Can you work these out from the model? Positions are in its coordinate system, mm. A direction names the side the tool comes from. Give positions to 0.01 mm unless a question says otherwise; leave off trailing zeros. Write each loop counter-clockwise with the first axis right and the second up, starting at its lowest first coordinate (ties: lowest second). Pieces come first, ordered by that corner, then holes. Notation, with made-up numbers: (23.5, -35) -> (73.5, -35) arc R11 cw to (73.5, -27) -> close; hole circle Ø1 at (73, 65.25). An arc over 180 degrees is marked (long way). One line per item, written item: value.
from build123d import *

# Parameters (mm, degrees)
SKETCH1_R                = 25
SKETCH1_R_2              = 22
BOSS_EXTRUDE2_DEPTH      = 2
BOSS_EXTRUDE2_DEPTH_BACK = 2
BOSS_EXTRUDE3_DEPTH      = 1.5
BOSS_EXTRUDE3_DEPTH_BACK = 1.5
BOSS_EXTRUDE5_DEPTH      = 0.5
BOSS_EXTRUDE5_DEPTH_BACK = 0.5


with BuildPart() as part:
    # Sketch1 → Boss-Extrude2 (new body, two sides)
    with BuildSketch(Plane(origin=(0, 0, 0), x_dir=(1, 0, 0), z_dir=(0, 1, 0))) as boss_extrude2_sk:
        Circle(SKETCH1_R)
        Circle(SKETCH1_R_2, mode=Mode.SUBTRACT)
    extrude(amount=BOSS_EXTRUDE2_DEPTH)
    extrude(boss_extrude2_sk.sketch, amount=-BOSS_EXTRUDE2_DEPTH_BACK)

    # Sketch1_5 → Boss-Extrude3 (add, two sides)
    with BuildSketch(Plane(origin=(0, 0, 0), x_dir=(1, 0, 0), z_dir=(0, 1, 0))) as boss_extrude3_sk:
        with BuildLine():
            Line((0, 22), (0, 4))
            ThreePointArc((0, 4), (-1.351805959, 3.764654121), (-2.544540937, 3.086310325))
            Line((-2.544540937, 3.086310325), (-13.994975151, 16.974706787))
            ThreePointArc((-13.994975151, 16.974706787), (-14.792671398, 16.284252298), (-15.556349186, 15.556349186))
            Line((-15.556349186, 15.556349186), (-2.828427125, 2.828427125))
            ThreePointArc((-2.828427125, 2.828427125), (-3.617883618, 1.706141297), (-3.981613111, 0.383088808))
            Line((-3.981613111, 0.383088808), (-21.89887211, 2.106988446))
            ThreePointArc((-21.89887211, 2.106988446), (-21.974703484, 1.054706969), (-22, 0))
            Line((-22, 0), (-4, 0))
            ThreePointArc((-4, 0), (-3.764654121, -1.351805959), (-3.086310325, -2.544540937))
            Line((-3.086310325, -2.544540937), (-16.974706787, -13.994975151))
            ThreePointArc((-16.974706787, -13.994975151), (-16.284252298, -14.792671398), (-15.556349186, -15.556349186))
            Line((-15.556349186, -15.556349186), (-2.828427125, -2.828427125))
            ThreePointArc((-2.828427125, -2.828427125), (-1.706141297, -3.617883618), (-0.383088808, -3.981613111))
            Line((-0.383088808, -3.981613111), (-2.106988446, -21.89887211))
            ThreePointArc((-2.106988446, -21.89887211), (-1.054706969, -21.974703484), (0, -22))
            Line((0, -22), (0, -4))
            ThreePointArc((0, -4), (1.351805959, -3.764654121), (2.544540937, -3.086310325))
            Line((2.544540937, -3.086310325), (13.994975151, -16.974706787))
            ThreePointArc((13.994975151, -16.974706787), (14.792671398, -16.284252298), (15.556349186, -15.556349186))
            Line((15.556349186, -15.556349186), (2.828427125, -2.828427125))
            ThreePointArc((2.828427125, -2.828427125), (3.617883618, -1.706141297), (3.981613111, -0.383088808))
            Line((3.981613111, -0.383088808), (21.89887211, -2.106988446))
            ThreePointArc((21.89887211, -2.106988446), (21.974703484, -1.054706969), (22, 0))
            Line((22, 0), (4, 0))
            ThreePointArc((4, 0), (3.764654121, 1.351805959), (3.086310325, 2.544540937))
            Line((3.086310325, 2.544540937), (16.974706787, 13.994975151))
            ThreePointArc((16.974706787, 13.994975151), (16.284252298, 14.792671398), (15.556349186, 15.556349186))
            Line((15.556349186, 15.556349186), (2.828427125, 2.828427125))
            ThreePointArc((2.828427125, 2.828427125), (1.706141297, 3.617883618), (0.383088808, 3.981613111))
            Line((0.383088808, 3.981613111), (2.106988446, 21.89887211))
            ThreePointArc((2.106988446, 21.89887211), (1.054706969, 21.974703484), (0, 22))
        make_face()
    extrude(amount=BOSS_EXTRUDE3_DEPTH)
    extrude(boss_extrude3_sk.sketch, amount=-BOSS_EXTRUDE3_DEPTH_BACK)

    # Sketch1_7 → Boss-Extrude5 (add, two sides)
    with BuildSketch(Plane(origin=(0, 0, 0), x_dir=(1, 0, 0), z_dir=(0, 1, 0))) as boss_extrude5_sk:
        with BuildLine():
            Line((2.106988446, 21.89887211), (0.383088808, 3.981613111))
            ThreePointArc((0.383088808, 3.981613111), (1.706141297, 3.617883618), (2.828427125, 2.828427125))
            Line((2.828427125, 2.828427125), (15.556349186, 15.556349186))
            ThreePointArc((15.556349186, 15.556349186), (9.383777136, 19.898359899), (2.106988446, 21.89887211))
        make_face()
        with BuildLine():
            ThreePointArc((6.167390973, 9.69056467), (4.235265266, 9.082555673), (3.459080714, 10.953470484))
            Line((3.459080714, 10.953470484), (5.375670734, 16.237642809))
            ThreePointArc((5.375670734, 16.237642809), (8.098483211, 17.367253291), (8.983341502, 14.555358302))
            Line((8.983341502, 14.555358302), (6.167390973, 9.69056467))
        make_face(mode=Mode.SUBTRACT)
        with BuildLine():
            ThreePointArc((-2.544540937, 3.086310325), (-1.351805959, 3.764654121), (0, 4))
            Line((0, 4), (0, 22))
            ThreePointArc((0, 22), (-7.434932773, 20.705597665), (-13.994975151, 16.974706787))
            Line((-13.994975151, 16.974706787), (-2.544540937, 3.086310325))
        make_face()
        with BuildLine():
            ThreePointArc((-2.491260012, 11.213267971), (-3.427551917, 9.417121496), (-5.299333827, 10.191212687))
            Line((-5.299333827, 10.191212687), (-7.680574112, 15.28292057))
            ThreePointArc((-7.680574112, 15.28292057), (-6.554010177, 18.006994968), (-3.940010864, 16.644374252))
            Line((-3.940010864, 16.644374252), (-2.491260012, 11.213267971))
        make_face(mode=Mode.SUBTRACT)
        with BuildLine():
            ThreePointArc((-3.981613111, 0.383088808), (-3.617883618, 1.706141297), (-2.828427125, 2.828427125))
            Line((-2.828427125, 2.828427125), (-15.556349186, 15.556349186))
            ThreePointArc((-15.556349186, 15.556349186), (-19.898359899, 9.383777136), (-21.89887211, 2.106988446))
            Line((-21.89887211, 2.106988446), (-3.981613111, 0.383088808))
        make_face()
        with BuildLine():
            ThreePointArc((-9.69056467, 6.167390973), (-9.082555673, 4.235265266), (-10.953470484, 3.459080714))
            Line((-10.953470484, 3.459080714), (-16.237642809, 5.375670734))
            ThreePointArc((-16.237642809, 5.375670734), (-17.367253291, 8.098483211), (-14.555358302, 8.983341502))
            Line((-14.555358302, 8.983341502), (-9.69056467, 6.167390973))
        make_face(mode=Mode.SUBTRACT)
        with BuildLine():
            ThreePointArc((-3.086310325, -2.544540937), (-3.764654121, -1.351805959), (-4, 0))
            Line((-4, 0), (-22, 0))
            ThreePointArc((-22, 0), (-20.705597665, -7.434932773), (-16.974706787, -13.994975151))
            Line((-16.974706787, -13.994975151), (-3.086310325, -2.544540937))
        make_face()
        with BuildLine():
            ThreePointArc((-11.213267971, -2.491260012), (-9.417121496, -3.427551917), (-10.191212687, -5.299333827))
            Line((-10.191212687, -5.299333827), (-15.28292057, -7.680574112))
            ThreePointArc((-15.28292057, -7.680574112), (-18.006994968, -6.554010177), (-16.644374252, -3.940010864))
            Line((-16.644374252, -3.940010864), (-11.213267971, -2.491260012))
        make_face(mode=Mode.SUBTRACT)
        with BuildLine():
            ThreePointArc((-0.383088808, -3.981613111), (-1.706141297, -3.617883618), (-2.828427125, -2.828427125))
            Line((-2.828427125, -2.828427125), (-15.556349186, -15.556349186))
            ThreePointArc((-15.556349186, -15.556349186), (-9.383777136, -19.898359899), (-2.106988446, -21.89887211))
            Line((-2.106988446, -21.89887211), (-0.383088808, -3.981613111))
        make_face()
        with BuildLine():
            ThreePointArc((-6.167390973, -9.69056467), (-4.235265266, -9.082555673), (-3.459080714, -10.953470484))
            Line((-3.459080714, -10.953470484), (-5.375670734, -16.237642809))
            ThreePointArc((-5.375670734, -16.237642809), (-8.098483211, -17.367253291), (-8.983341502, -14.555358302))
            Line((-8.983341502, -14.555358302), (-6.167390973, -9.69056467))
        make_face(mode=Mode.SUBTRACT)
        with BuildLine():
            Line((21.89887211, -2.106988446), (3.981613111, -0.383088808))
            ThreePointArc((3.981613111, -0.383088808), (3.617883618, -1.706141297), (2.828427125, -2.828427125))
            Line((2.828427125, -2.828427125), (15.556349186, -15.556349186))
            ThreePointArc((15.556349186, -15.556349186), (19.898359899, -9.383777136), (21.89887211, -2.106988446))
        make_face()
        with BuildLine():
            ThreePointArc((9.69056467, -6.167390973), (9.082555673, -4.235265266), (10.953470484, -3.459080714))
            Line((10.953470484, -3.459080714), (16.237642809, -5.375670734))
            ThreePointArc((16.237642809, -5.375670734), (17.367253291, -8.098483211), (14.555358302, -8.983341502))
            Line((14.555358302, -8.983341502), (9.69056467, -6.167390973))
        make_face(mode=Mode.SUBTRACT)
        with BuildLine():
            Line((13.994975151, -16.974706787), (2.544540937, -3.086310325))
            ThreePointArc((2.544540937, -3.086310325), (1.351805959, -3.764654121), (0, -4))
            Line((0, -4), (0, -22))
            ThreePointArc((0, -22), (7.434932773, -20.705597665), (13.994975151, -16.974706787))
        make_face()
        with BuildLine():
            ThreePointArc((2.491260012, -11.213267971), (3.427551917, -9.417121496), (5.299333827, -10.191212687))
            Line((5.299333827, -10.191212687), (7.680574112, -15.28292057))
            ThreePointArc((7.680574112, -15.28292057), (6.554010177, -18.006994968), (3.940010864, -16.644374252))
            Line((3.940010864, -16.644374252), (2.491260012, -11.213267971))
        make_face(mode=Mode.SUBTRACT)
        with BuildLine():
            Line((16.974706787, 13.994975151), (3.086310325, 2.544540937))
            ThreePointArc((3.086310325, 2.544540937), (3.764654121, 1.351805959), (4, 0))
            Line((4, 0), (22, 0))
            ThreePointArc((22, 0), (20.705597665, 7.434932773), (16.974706787, 13.994975151))
        make_face()
        with BuildLine():
            ThreePointArc((11.213267971, 2.491260012), (9.417121496, 3.427551917), (10.191212687, 5.299333827))
            Line((10.191212687, 5.299333827), (15.28292057, 7.680574112))
            ThreePointArc((15.28292057, 7.680574112), (18.006994968, 6.554010177), (16.644374252, 3.940010864))
            Line((16.644374252, 3.940010864), (11.213267971, 2.491260012))
        make_face(mode=Mode.SUBTRACT)
    extrude(amount=BOSS_EXTRUDE5_DEPTH)
    extrude(boss_extrude5_sk.sketch, amount=-BOSS_EXTRUDE5_DEPTH_BACK)


solid = part.part
1) Will these pins go through, and if not, where does the flat tip stop? pin 1 (3.5 mm diameter, centred on x = 15.56, z = 7.25, fed in from +Y); pin 2 (7.5 mm diameter, centred on x = -7, z = 8, fed in from -Y); pin 3 (2 mm diameter, centred on x = 2.5, z = 10.5, fed in from +Y); pin 4 (0.8 mm diameter, centred on y = -1, z = -15, fed in from -X).
Answer list:
pin 1: passes through
pin 2: stops at y = -1.5
pin 3: stops at y = 0.5
pin 4: stops at x = -20.29
2) For faces 1 (the face through (-9.933, -0.993, 8.19)), 2 (the face through (-8, 0.5, 12)), 3 (the face through (-13.967, 0.007, 3.226)), which set-ups out of +Z, -Z, +X, -X, +Y, -Y let a thin tool reach every point of the face, with its end or its side?
Answer list:
face 1: -Y
face 2: +Y
face 3: +Y, -Y
3) If we section it at A-A (x = -19): Write out the boundary of the cut face in (y, z).
Answer list:
outline: (-2, -16.25) -> (2, -16.25) -> (2, -11.09) -> (0.5, -11.09) -> (0.5, -1.83) -> (1.5, -1.83) -> (1.5, 0) -> (0.5, 0) -> (0.5, 11.09) -> (2, 11.09) -> (2, 16.25) -> (-2, 16.25) -> (-2, 11.09) -> (-0.5, 11.09) -> (-0.5, 0) -> (-1.5, 0) -> (-1.5, -1.83) -> (-0.5, -1.83) -> (-0.5, -11.09) -> (-2, -11.09) -> close
4) If we section it at B-B (z = -12.5): State how many separate pieces and enclosed holes the cut face has, and give its area (3 significant figures).
Answer list:
separate pieces: 3
enclosed holes: 0
area: 69.4 mm^2
5) I need wall thicknesses on L1, parallel to X at y = 0.7, z = -12.5; L2, parallel to X at y = -1.3, z = 14.5; L3, parallel to Z at x = 7, y = -0.6. Which ranges of each line are inside material? Lowest first, please.
Answer list:
L1: x = -21.65 to -18.1, -12.5 to -10.31, 0 to 1.2, 12.5 to 15.16, 18.1 to 21.65
L2: x = -20.37 to -14.5, -1.4 to 0, 11.95 to 14.5, 16.55 to 20.37
L3: z = -24 to -20.86, -7 to -5.77, 0 to 0.67, 7 to 8.49, 20.86 to 24
